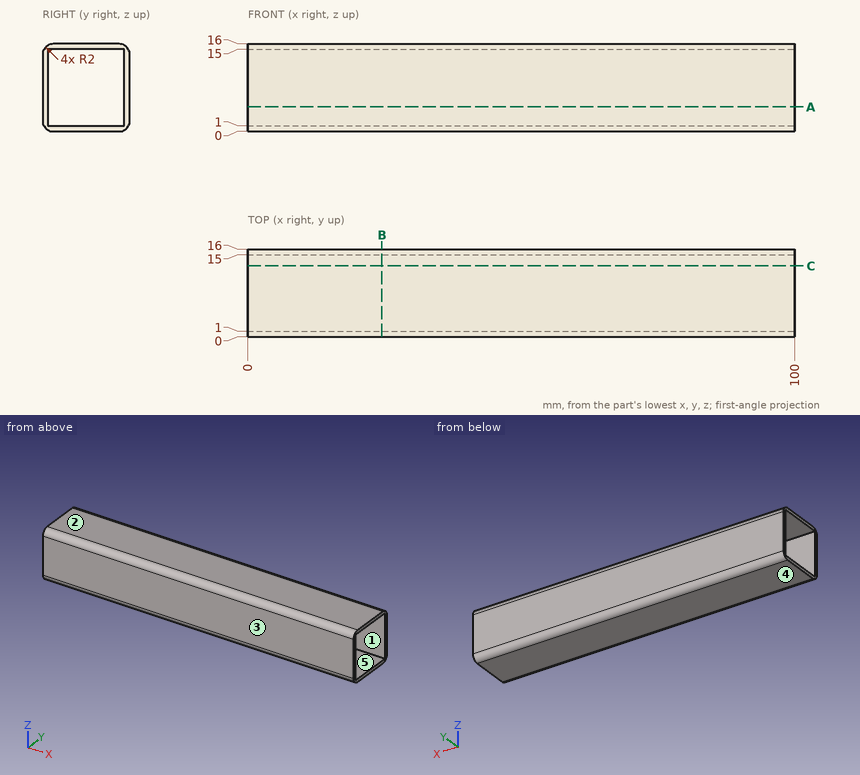
Source: three-view drawing plus pictorial views. Frame: mm from the lowest corner of the part. A direction names the side the tool comes from. Give positions to 0.01 mm unless a question says otherwise; leave off trailing zeros. Order: outer loops, then holes, each group sorted by start corner. A loop starts at its lowest first (then second) coordinate and runs counter-clockwise, first axis right, second up. Notation, with made-up numbers: (-7, 73) - (-3, 73) arc R27 cw to (-3, 98) - close; hole circle Ø6 at (49.5, 29.25). An arc over 180 degrees is marked (long way). Put each result on its own line as item: value.
Item 1: Ray query, L1, parallel to Z at x = 54, y = 12; L2, parallel to Z at x = 54.5, y = 14.5. Return the intervals inside material, ascending. Write a range as from..to.
Found:
L1: z = 0..1, 15..16
L2: z = 0.06..1, 15..15.94
Item 2: Access query for the marked faces 4 and 5. Directions: +Z, -Z, +X, -X, +Y, -Y. A direction counts if a zero-diameter tool reaches every point of the face in a straight line with its end or side. Return the directions, or none.
Found:
face 4: -Z, +X, -X, +Y, -Y
face 5: +X, -X
Item 3: Section query B-B, the plane x = 24.5. Return loops of the section in (y, z), then the cut area to 3 significant figures.
Found:
outline: (0, 2) arc R2 ccw to (2, 0) - (14, 0) arc R2 ccw to (16, 2) - (16, 14) arc R2 ccw to (14, 16) - (2, 16) arc R2 ccw to (0, 14) - close; hole (1, 1) - (15, 1) - (15, 15) - (1, 15) - close
area: 56.6 mm^2
Item 4: Section query A-A, the plane z = 4.5. Return loops of the section in (x, y), then the cut area to 3 significant figures.
Found:
outline: (0, 0) - (100, 0) - (100, 1) - (0, 1) - close; (0, 15) - (100, 15) - (100, 16) - (0, 16) - close
area: 200 mm^2
Item 5: Draft query along Z for the marked faces 1, 2 and 3. Return one class per face: +Z half, -Z half, draft (parallel to the pull), parting line (faces both ways), or undercut.
Found:
face 1: undercut
face 2: +Z half
face 3: draft
